Part model, mm, in its own coordinate system. Give positions to 0.01 mm unless a question says otherwise; leave off trailing zeros. Order: outer loops, then holes, each group sorted by start corner. A loop starts at its lowest first (then second) coordinate and runs counter-clockwise, first axis right, second up. Notation, with made-up numbers: M -28,80.25 L 1,80.25 A28 ccw 1,110.25 Z; hole C -21.5,-22 d6. An arc over 180 degrees is marked long. One line per question, with ' | ' between items.
```python
from build123d import *

# Parameters (mm, degrees)
SKETCH1_W           = 140
SKETCH1_H           = 200
BOSS_EXTRUDE1_DEPTH = 3
SKETCH2_R           = 2.5
CUT_EXTRUDE1_DEPTH  = 10
SKETCH3_W           = 3
SKETCH3_H           = 10
CUT_EXTRUDE2_DEPTH  = 10


with BuildPart() as part:
    # Sketch1 → Boss-Extrude1 (new body)
    with BuildSketch(Plane(origin=(0, 0, 0), x_dir=(1, 0, 0), z_dir=(0, 1, 0))):
        Rectangle(SKETCH1_W, SKETCH1_H)
    extrude(amount=BOSS_EXTRUDE1_DEPTH)

    # Sketch2 → Cut-Extrude1 (cut)
    with BuildSketch(Plane(origin=(0, 3, 0), x_dir=(1, 0, 0), z_dir=(0, 1, 0))):
        with Locations(Location((-30, 40, 0), (0, 0, 270))):
            Circle(SKETCH2_R)
        with Locations(Location((30, 40, 0), (0, 0, 270))):
            Circle(SKETCH2_R)
        with Locations(Location((-30, -40, 0), (0, 0, 270))):
            Circle(SKETCH2_R)
        with Locations(Location((30, -40, 0), (0, 0, 270))):
            Circle(SKETCH2_R)
    extrude(amount=-CUT_EXTRUDE1_DEPTH, mode=Mode.SUBTRACT)

    # Sketch3 → Cut-Extrude2 (cut)
    with BuildSketch(Plane(origin=(0, 3, 0), x_dir=(1, 0, 0), z_dir=(0, 1, 0))):
        with Locations((68.5, -45)):
            Rectangle(SKETCH3_W, SKETCH3_H)
        with Locations((68.5, -75)):
            Rectangle(SKETCH3_W, SKETCH3_H)
        with Locations((68.5, -15)):
            Rectangle(SKETCH3_W, SKETCH3_H)
        with Locations((68.5, 15)):
            Rectangle(SKETCH3_W, SKETCH3_H)
        with Locations((68.5, 45)):
            Rectangle(SKETCH3_W, SKETCH3_H)
        with Locations((68.5, 75)):
            Rectangle(SKETCH3_W, SKETCH3_H)
        with Locations((-68.5, -75)):
            Rectangle(SKETCH3_W, SKETCH3_H)
        with Locations((-68.5, -45)):
            Rectangle(SKETCH3_W, SKETCH3_H)
        with Locations((-68.5, -15)):
            Rectangle(SKETCH3_W, SKETCH3_H)
        with Locations((-68.5, 15)):
            Rectangle(SKETCH3_W, SKETCH3_H)
        with Locations((-68.5, 45)):
            Rectangle(SKETCH3_W, SKETCH3_H)
        with Locations((-68.5, 75)):
            Rectangle(SKETCH3_W, SKETCH3_H)
    extrude(amount=-CUT_EXTRUDE2_DEPTH, mode=Mode.SUBTRACT)


solid = part.part
```
1. Probe L1, parallel to X at y = 0.75, z = -39; L2, parallel to Z at x = -32, y = 0.25; L3, parallel to X at y = 2.8, z = -77. List the from-to ranges inside material, lowest first. Write a range as from..to.
Worked out:
L1: x = -70..-32.29, -27.71..27.71, 32.29..70 | L2: z = -100..-41.5, -38.5..38.5, 41.5..100 | L3: x = -67..67
2. Slice it at A-A on x = 30. Give the cut face in (y, z).
Worked out:
outline: M 0,-100 L 3,-100 L 3,-42.5 L 0,-42.5 Z; M 0,-37.5 L 3,-37.5 L 3,37.5 L 0,37.5 Z; M 0,42.5 L 3,42.5 L 3,100 L 0,100 Z
3. Slice it at B-B on y = 0.8. Give the number of separate pieces and of enclosed holes in the cut face, then the cut area to 3 significant figures.
Worked out:
separate pieces: 1 | enclosed holes: 4 | area: 27,600 mm2
4. Slice it at C-C on z = -48. Give the cut face in (x, y).
Worked out:
outline: M -67,0 L 67,0 L 67,3 L -67,3 Z
5. Drop flat-ended pins along their axis: pin 1 (0.9 mm diameter, centred on y = 1, z = 17, fed in from -X); pin 2 (8 mm diameter, centred on x = 30, z = 40, fed in from -Y); pin 3 (1.5 mm diameter, centred on y = 1.5, z = 17.5, fed in from +X). Give the stop position or say it passes through.
Worked out:
pin 1: stops at x = -67 | pin 2: stops at y = 0 | pin 3: stops at x = 67
6. Mould opens along X. For faces 1 (the cylindrical face through (32.11, 1.52, -38.66)), 2 (the flat face through (-1, 0, -1)), 3 (the cylindrical face through (-27.89, 1.52, 41.34)) say: released by +X, released by -X, zero draft, split by the parting line, or undercut.
Worked out:
face 1: undercut | face 2: zero draft | face 3: undercut
